Part model, mm, in its own coordinate system. A direction names the side the tool comes from. Round coordinates to 2 decimals unless told otherwise and drop trailing zeros. Loops run counter-clockwise (first coordinate to the right, second up) from the corner with the lowest first, then second, coordinate; pieces in that order, holes last.
1) 3-axis set-ups, long thin cutter, end or side, ignore diameter. For faces 4 (the flat face through (-10, 10, 20)), 5 (the flat face through (-30, 10, 15)), 6 (the flat face through (-30, 10, -15)): which of +Z, -Z, +X, -X, +Y, -Y reach the whole face in a straight line?
2) Drop flat-ended pins along their axis: P1, Ø8, axis at y = 13.5, z = -15.5, coming from the +X side; P2, Ø12, axis at y = 11, z = 11, coming from the +X side; P3, Ø5, axis at x = -26.5, y = 12.5, coming from the +Z side. Give the stop position or say it passes through.
3) Mould opens along X. For faces 1 (the flat face through (-40, 10, -20)), 2 (the cylindrical face through (20, 10, 0)), 3 (the flat face through (-20, 10, -15)) say: +X half, -X half, draft (parallel to the pull), parting line (faces both ways), or undercut.
4) Band-saw the part on C-C, the plane x = 4.5. Write the cut outline in (y, z), then the cut area to 3 significant figures.
5) Band-saw the part on A-A, the plane z = 12. Write the cut outline in (x, y).
6) Probe line 1 (X direction, y = 13, z = 0); line 2 (Z direction, x = 0, y = 12); line 3 (X direction, y = 11.75, z = 8.5). List the from-to ranges inside material, lowest first.
7) Band-saw the part on B-B, the plane y = 4.5. Write the cut outline in (x, z), then the cut area to 3 significant figures.
Autodesk Inventor part; units mm, degrees
ref_plane "YZ Plane" through (0, 0, 0) normal (1, 0, 0) x (0, 1, 0)
ref_plane "XZ Plane" through (0, 0, 0) normal (0, 1, 0) x (-1, 0, 0)
ref_plane "XY Plane" through (0, 0, 0) normal (0, 0, 1) x (1, 0, 0)
sketch "草圖1" plane through (0, 0, 0) normal (0, 1, 0) x (-1, 0, 0)
  circle A0 centre (0, 0) radius 20
  line L0 (0, -20) -> (50, -20)
  line L1 (50, -20) -> (50, 20)
  line L2 (50, 20) -> (0, 20)
  line L3 (0, 20) -> (0, -20)
  point P0 (0, 20)
  dimension "d0" = 40
  dimension "d1" = 50
extrude "擠出1" add sketch "草圖1" along normal blind 20
sketch "草圖2" plane through (0, 20, 0) normal (0, 1, 0) x (1, 0, 0)
  line L0 (-50, -20) -> (-50, 20)
  line L1 (-50, 20) -> (0, 20)
  arc A0 (0, -20) -> (0, 20) centre (0, 0) ccw
  line L2 (0, -20) -> (-50, -20)
  line L3 (-30, -10) -> (-20, -10)
  line L4 (-20, -10) -> (-20, -20)
  line L5 (-20, -20) -> (-30, -20)
  line L6 (-30, -20) -> (-30, -10)
  line L7 (-50, -20) -> (0, -20)
  dimension "d4" = 10
  dimension "d5" = 10
  dimension "d6" = 20
extrude "擠出2" cut sketch "草圖2" against normal through all contours L6 L3 L4 L2
mirror "鏡射1" about plane through (0, 0, 0) normal (0, 0, 1) of "擠出2"
sketch "草圖3" plane through (0, 20, 0) normal (0, 1, 0) x (1, 0, 0)
  arc A0 (0, -20) -> (0, 20) centre (0, 0) ccw
hole "孔1" at (0, 20, 0) direction (0, -1, 0) diameter 20 end through all
properties part number "32" material "鋼、碳鋼"
Reported:
1. face 4: +Z, +X, -X, +Y, -Y
1. face 5: +Z, +Y, -Y
1. face 6: -Z, +Y, -Y
2. P1: stops at x = 16.36
2. P2: stops at x = 19.36
2. P3: stops at z = 10
3. face 1: draft
3. face 2: +X half
3. face 3: undercut
4. outline: (0, -19.49) - (20, -19.49) - (20, -8.93) - (0, -8.93) - close; (0, 8.93) - (20, 8.93) - (20, 19.49) - (0, 19.49) - close
4. area: 422 mm2
5. outline: (-50, 0) - (-30, 0) - (-30, 20) - (-50, 20) - close; (-20, 0) - (16, 0) - (16, 20) - (-20, 20) - close
6. line 1: x = -50 to -10, 10 to 20
6. line 2: z = -20 to -10, 10 to 20
6. line 3: x = -50 to -5.27, 5.27 to 18.1
7. outline: (-50, -20) - (-30, -20) - (-30, -10) - (-20, -10) - (-20, -20) - (0, -20) arc R20 ccw to (0, 20) - (-20, 20) - (-20, 10) - (-30, 10) - (-30, 20) - (-50, 20) - close; hole circle Ø20 at (0, 0)
7. area: 2,110 mm2
